Can you work these out from the model? Positions are in its coordinate system, mm. Face numbers are marked on the shaded views. A direction names the side the tool comes from. Give positions to 0.01 mm unless a question says otherwise; leave off trailing zeros. Loops run counter-clockwise (first coordinate to the right, second up) from the corner with the lowest first, then second, coordinate; pieces in that order, holes last. Notation, with made-up numbers: (-40, 89.25) - (-27, 89.25) arc R3 ccw to (-27, 93.25) - close; hole circle Ø2 at (58.25, -4). An arc over 180 degrees is marked (long way). Answer as a JSON object with one key per item and string values. Group by question number.
Item 1: Will these pins go through, and if not, where does the flat tip stop? pin 1 (4 mm diameter, centred on x = -250.5, y = 20, fed in from +Z); pin 2 (6 mm diameter, centred on y = 14.5, z = 67.5, fed in from -X); pin 3 (10.5 mm diameter, centred on x = 25.4, z = 25.4, fed in from -Y); pin 4 (8.5 mm diameter, centred on y = 8, z = 68.5, fed in from +X).
Item 2: Suppose I cut it at B-B on z = -53. Write out the boundary of the cut face in (x, y).
Item 3: Suppose I cut it at D-D on y = 73.5. Write out the boundary of the cut face in (x, z).
Item 4: Which directions (+Z, -Z, +X, -X, +Y, -Y) give clear straight access to the entire face, cutting with the end or side of a thin tool? Please do the marked faces 1 and 2.
Item 5: Suppose I cut it at A-A on y = 50. Write out the boundary of the cut face in (x, z).
Item 6: Please list where these lines run through material, in increasing order: L1, parallel to X at y = 13.5, z = -3; L2, parallel to Y at x = -255, z = -44; L3, parallel to Y at x = 124.5, z = 28.
Item 7: Thinking about a two-plate mould opening in X: for the marked faces 3, 4, 5 and 6, which applies, pulls with the +X half, pulls with the -X half, needs draft (parallel to the pull), parting line crosses it, or undercut?
Item 8: Suppose I cut it at C-C on x = 184.5. Write out the boundary of the cut face in (y, z).
from build123d import *

# Parameters (mm, degrees)
SKETCH1_W                      = 511.175
SKETCH1_H                      = 127
BASE_FLANGE1_DEPTH             = 1.42875
EDGE_FLANGE1_STRIP_W           = 18.415
EDGE_FLANGE1_STRIP_H           = 1.42875
EDGE_FLANGE1_STRIP_CUT_DEPTH   = 127
EDGE_FLANGE1_STRIP_2_W         = 18.415
EDGE_FLANGE1_STRIP_2_H         = 1.42875
EDGE_FLANGE1_STRIP_CUT_2_DEPTH = 127
EDGE_FLANGE1_DEPTH             = 127
EDGE_FLANGE1_BEND_DEPTH        = 127
CUT_EXTRUDE1_DEPTH             = 534.339544007
FILLET1_R                      = 31.75
SKETCH14_R                     = 14.224
CUT_EXTRUDE2_DEPTH             = 534.339544007
H_0_266_DIAMETER_HOLE1_D       = 6.7564
F_0_257_DIAMETER_HOLE2_D       = 6.5278
EDGE_FLANGE2_DEPTH             = 495.6175


# Sheet-metal steps are written as plain solids
with BuildPart() as part:
    # Sketch1 → Base-Flange1 (new body)
    with BuildSketch(Plane(origin=(0, 0, 0), x_dir=(1, 0, 0), z_dir=(0, 1, 0))):
        Rectangle(SKETCH1_W, SKETCH1_H)
    extrude(amount=-BASE_FLANGE1_DEPTH)

    # Edge-Flange1 strip (across the edge) → Edge-Flange1 strip cut (cut)
    with BuildSketch(Plane(origin=(255.5875, 0, 63.5), x_dir=(-1, 0, 0), z_dir=(0, 0, -1))):
        with Locations((-1.42875, -0.714375)):
            Rectangle(EDGE_FLANGE1_STRIP_W, EDGE_FLANGE1_STRIP_H)
    extrude(amount=EDGE_FLANGE1_STRIP_CUT_DEPTH, mode=Mode.SUBTRACT)

    # Edge-Flange1 strip 2 (across the edge) → Edge-Flange1 strip cut 2 (cut)
    with BuildSketch(Plane(origin=(-255.5875, 0, -63.5), x_dir=(1, 0, 0), z_dir=(0, 0, 1))):
        with Locations((-1.42875, -0.714375)):
            Rectangle(EDGE_FLANGE1_STRIP_2_W, EDGE_FLANGE1_STRIP_2_H)
    extrude(amount=EDGE_FLANGE1_STRIP_CUT_2_DEPTH, mode=Mode.SUBTRACT)

    # Edge-Flange1 section (across the edge) → Edge-Flange1 (add)
    with BuildSketch(Plane(origin=(255.5875, 0, 63.5), x_dir=(-1, 0, 0), z_dir=(0, 0, -1))):
        with BuildLine():
            Line((0, 6.35), (0, 138.27125))
            Line((0, 138.27125), (1.42875, 138.27125))
            Line((1.42875, 138.27125), (1.42875, 6.35))
            ThreePointArc((1.42875, 6.35), (3.288621939, 1.859871939), (7.77875, 0))
            Line((7.77875, 0), (7.77875, -1.42875))
            ThreePointArc((7.77875, -1.42875), (2.278343126, 0.849593126), (0, 6.35))
        make_face()
    extrude(amount=EDGE_FLANGE1_DEPTH)

    # Edge-Flange1 section 2 (across the edge) → Edge-Flange1 bend (add)
    with BuildSketch(Plane(origin=(-255.5875, 0, -63.5), x_dir=(1, 0, 0), z_dir=(0, 0, 1))):
        with BuildLine():
            Line((0, 6.35), (0, 138.27125))
            Line((0, 138.27125), (1.42875, 138.27125))
            Line((1.42875, 138.27125), (1.42875, 6.35))
            ThreePointArc((1.42875, 6.35), (3.288621939, 1.859871939), (7.77875, 0))
            Line((7.77875, 0), (7.77875, -1.42875))
            ThreePointArc((7.77875, -1.42875), (2.278343126, 0.849593126), (0, 6.35))
        make_face()
    extrude(amount=EDGE_FLANGE1_BEND_DEPTH)

    # Sketch13 → Cut-Extrude1 (cut, through all)
    with BuildSketch(Plane(origin=(255.5875, 0, 0), x_dir=(0, 0, -1), z_dir=(1, 0, 0))):
        Polygon((-63.5, 36.67125), (0, 138.27125), (-63.5, 138.27125), align=None)
    extrude(amount=-CUT_EXTRUDE1_DEPTH, mode=Mode.SUBTRACT)

    # Fillet1
    fillet1_edges = [part.edges().sort_by_distance(p)[0] for p in [
        (254.873125, 138.27125, -63.5),
        (-254.873125, 138.27125, -63.5),
        (254.873125, 138.27125, 0),
        (254.873125, 36.67125, 63.5),
        (-254.873125, 138.27125, 0),
        (-254.873125, 36.67125, 63.5),
    ]]
    fillet(fillet1_edges, radius=FILLET1_R)

    # Sketch14 → Cut-Extrude2 (cut, through all)
    with BuildSketch(Plane(origin=(255.5875, 0, 0), x_dir=(0, 0, -1), z_dir=(1, 0, 0))):
        with Locations(Location((31.75, 106.52125, 0), (0, 0, 90))):
            Circle(SKETCH14_R)
    extrude(amount=-CUT_EXTRUDE2_DEPTH, mode=Mode.SUBTRACT)

    # H (0.266) Diameter Hole1 (through all)
    with Locations(Plane(origin=(255.5875, 0, 0), x_dir=(0, 0, -1), z_dir=(1, 0, 0))):
        with Locations((-44.45, 17.62125), (44.45, 17.62125)):
            Hole(H_0_266_DIAMETER_HOLE1_D / 2)

    # F (0.257) Diameter Hole2 (through all)
    with Locations(Plane(origin=(0, 0, 0), x_dir=(1, 0, 0), z_dir=(0, 1, 0))):
        with Locations((-25.4, -25.4), (25.4, -25.4)):
            Hole(F_0_257_DIAMETER_HOLE2_D / 2)

    # Edge-Flange2 section (across the edge) → Edge-Flange2 (add)
    with BuildSketch(Plane(origin=(-247.80875, 0, 69.85), x_dir=(0, 0, -1), z_dir=(1, 0, 0))):
        with BuildLine():
            Line((-1.42875, 6.35), (-1.42875, 25.4))
            Line((-1.42875, 25.4), (0, 25.4))
            Line((0, 25.4), (0, 6.35))
            ThreePointArc((0, 6.35), (1.859871939, 1.859871939), (6.35, 0))
            Line((6.35, 0), (6.35, -1.42875))
            ThreePointArc((6.35, -1.42875), (0.849593126, 0.849593126), (-1.42875, 6.35))
        make_face()
    extrude(amount=EDGE_FLANGE2_DEPTH)


solid = part.part
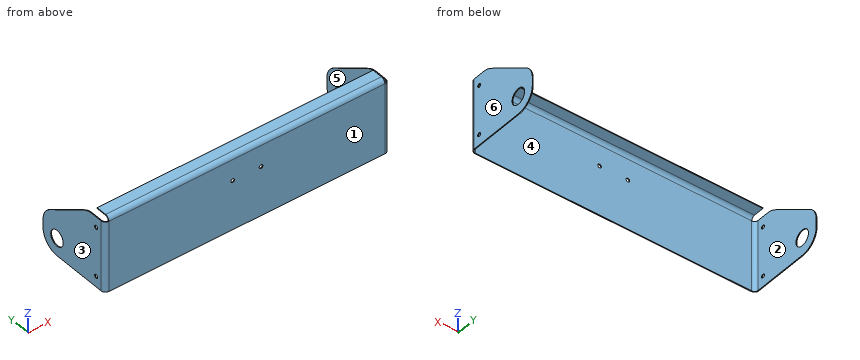
Worked out:
{
 "1": {"pin 1": "passes through", "pin 2": "stops at x = -247.81", "pin 3": "stops at y = -1.43", "pin 4": "stops at x = 247.81"},
 "2": {"outline": "(-255.59, 6.35) arc R7.78 ccw to (-247.81, -1.43) - (247.81, -1.43) arc R7.78 ccw to (255.59, 6.35) - (255.59, 130.11) - (254.16, 130.11) - (254.16, 6.35) arc R6.35 cw to (247.81, 0) - (-247.81, 0) arc R6.35 cw to (-254.16, 6.35) - (-254.16, 130.11) - (-255.59, 130.11) - close"},
 "3": {"outline": "(-255.59, -63.5) - (-254.16, -63.5) - (-254.16, 40.48) - (-255.59, 40.48) - close; (254.16, -63.5) - (255.59, -63.5) - (255.59, 40.48) - (254.16, 40.48) - close"},
 "4": {"face 1": "+Z, -Z, +X, -X, -Y", "face 2": "+Z, -Z, +Y"},
 "5": {"outline": "(-255.59, -63.5) - (-254.16, -63.5) - (-254.16, 55.17) - (-255.59, 55.17) - close; (254.16, -63.5) - (255.59, -63.5) - (255.59, 55.17) - (254.16, 55.17) - close"},
 "6": {"L1": "x = -255.59 to -254.16, 254.16 to 255.59", "L2": "y = 3.38 to 14.27, 20.97 to 99.29, 113.75 to 135.81", "L3": "y = -1.43 to 0"},
 "7": {"face 3": "pulls with the -X half", "face 4": "undercut", "face 5": "undercut", "face 6": "pulls with the +X half"},
 "8": {"outline": "(-1.43, -63.5) - (0, -63.5) - (0, 63.5) arc R6.35 cw to (6.35, 69.85) - (25.4, 69.85) - (25.4, 71.28) - (6.35, 71.28) arc R7.78 ccw to (-1.43, 63.5) - close"}
}
